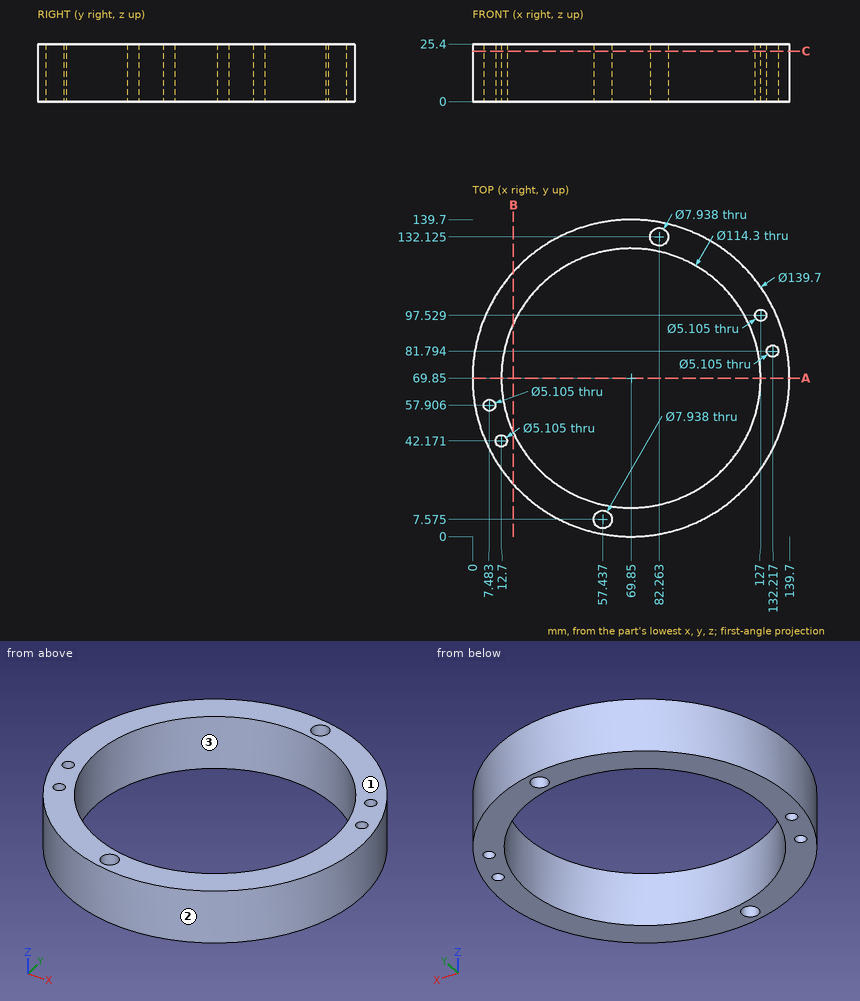
Geometry check sheet. Reference: drawing and pictorial views, mm from the part's lowest x, y, z. Round coordinates to 2 decimals unless told otherwise and drop trailing zeros. Order: outer loops, then holes, each group sorted by start corner. A loop starts at its lowest first (then second) coordinate and runs counter-clockwise, first axis right, second up.
Q1. Cross-section at A-A, the plane y = 69.85. Enter the section's corners in (x, z), plus the area to 3 significant figures.
Filled sheet:
outline: (0, 0) - (12.7, 0) - (12.7, 25.4) - (0, 25.4) - close; (127, 0) - (139.7, 0) - (139.7, 25.4) - (127, 25.4) - close
area: 645 mm2
Q2. Depth check by flat-ended pin: P1, Ø2, axis at x = 74, z = 20.5, coming from the -Y side; P2, Ø2, axis at x = 113, z = 21.5, coming from the +Y side; P3, Ø10, axis at y = 51, z = 16.5, coming from the -X side. Enter the tip coordinate at first touch or a pass-through.
Filled sheet:
P1: stops at y = 0.07
P2: stops at y = 125.55
P3: stops at x = 1.39
Q3. Scan lines: L1, parallel to Y at x = 70.5, z = 15.25; L2, parallel to Y at x = 35, z = 9.5 (1 decimal); L3, parallel to X at y = 64, z = 4 (1 decimal). Record each from-to range of solid material in increasing order.
Filled sheet:
L1: y = 0 to 12.7, 127 to 139.7
L2: y = 9.3 to 24.6, 115.1 to 130.4
L3: x = 0.2 to 13, 126.7 to 139.5
Q4. Cross-section at C-C, the plane z = 22.25. Give the number of separate pieces and of enclosed holes in the cut face, plus the area to 3 significant figures.
Filled sheet:
separate pieces: 1
enclosed holes: 7
area: 4,890 mm2
Q5. Cross-section at B-B, the plane x = 18. Enter the section's corners in (y, z) (1 decimal).
Filled sheet:
outline: (23, 0) - (45.8, 0) - (45.8, 25.4) - (23, 25.4) - close; (93.9, 0) - (116.7, 0) - (116.7, 25.4) - (93.9, 25.4) - close
Q6. Draft check along Y on the marked faces 1, 2 and 3. Enter one of: pulls with the +Y half, pulls with the -Y half, needs draft (parallel to the pull), parting line crosses it, or undercut.
Filled sheet:
face 1: needs draft
face 2: parting line crosses it
face 3: undercut
